Autodesk Inventor part; units mm, degrees
ref_plane "Work Plane4" through (-32.48, 0, 0) normal (1, 0, 0) x (0, 1, 0)
ref_plane "Work Plane5" through (30.48, 0, 0) normal (1, 0, 0) x (0, 1, 0)
ref_plane "XZ Plane" through (0, 0, 0) normal (0, 1, 0) x (-1, 0, 0)
sketch "Sketch1" plane through (0, 0, 0) normal (0, 1, 0) x (-1, 0, 0)
  circle A0 centre (0, 0) radius 30.48
  circle A1 centre (0, 0) radius 32.48
  dimension "d0" = 60.96
  dimension "d2" = 2
extrude "Extrusion1" add sketch "Sketch1" along normal blind 19.05
sketch "Sketch2" plane through (0, 19.05, 0) normal (0, 1, 0) x (1, 0, 0)
  circle A0 centre (0, 0) radius 32.48
  circle A1 centre (0, 0) radius 32.48
extrude "Extrusion2" add sketch "Sketch2" along normal blind 12.7
fillet "Fillet1" radius 6.35 1 edges at (-32.48, 31.75, 0)
sketch "Sketch6" plane through (0, 31.75, 0) normal (0, 1, 0) x (1, 0, 0)
  circle A0 centre (0, 0) radius 3.302
  dimension "d15" = 6.604
extrude "Extrusion5" cut sketch "Sketch6" against normal up to surface (12.7 mm away)
sketch "Sketch10" plane through (0, 0, 0) normal (0, 0, 1) x (1, 0, 0)
  line L0 (-17.78, 19.05) -> (-17.78, -12.7)
  line L1 (-17.78, -12.7) -> (-25.4, -12.7)
  line L2 (-25.4, -12.7) -> (-25.4, 19.05)
  line L3 (-17.78, 19.05) -> (-25.4, 19.05)
  line L4 (-26.13, 31.75) -> (26.13, 31.75)
  line L5 (0, 31.75) -> (0, 0)
  line L6 (32.48, 0) -> (-32.48, 0)
  line L7 (-30.48, 0) -> (-30.48, 19.05)
  line L8 (-17.78, -12.7) -> (-25.4, -8.3006)
  line L9 (-30.48, 19.05) -> (30.48, 19.05)
  point P0 (-30.48, 0)
  point P1 (-25.4, 19.05)
  dimension "d29" = 7.62
  dimension "d33" = 30
  dimension "d42" = 25.4
  dimension "d89" = 31.75
revolve "Revolution2" add sketch "Sketch10" angle 360 about axis through (0, 31.75, 0) along (0, -1, 0) contours L0 L6 L2 L3 | L0 L8 L2 L6
sketch "Sketch11" plane through (0, 0, 0) normal (0, 0, 1) x (1, 0, 0)
  line L0 (25.4, -7.0306) -> (25.4, 25.4)
  circle A0 centre (26.3462, -3.81) radius 2.3813
  circle A1 centre (26.3462, 2.54) radius 2.3813
  line L1 (0, -11.43) -> (0, 31.75)
  line L2 (-26.13, 31.75) -> (26.13, 31.75)
  line L3 (26.3462, 2.54) -> (26.3462, -3.81)
  line L4 (30.48, 19.05) -> (30.48, 0)
  line L5 (30.48, 0) -> (29.972, 19.05)
  line L6 (29.972, 19.05) -> (29.972, 0)
  line L7 (-25.4, -5.08) -> (25.4, -5.08)
  line L8 (-17.78, -12.7) -> (17.78, -12.7)
  point P0 (0, 0)
  point P1 (25.4, -8.3006)
  point P2 (27.772, -0.6806)
  point P3 (17.78, -12.7)
  dimension "d36" = 6.35
  dimension "d37" = 4.7625
  dimension "d38" = 4.7625
  dimension "d43" = 26.3462
  dimension "d91" = 8.89
revolve "Revolution3" cut sketch "Sketch11" angle 360 about axis through (0, -11.43, 0) along (0, 1, 0) contours A0 L7 L0 | L0 A0 | L7 A0 L0 | A1 L0 | L0 A1
sketch "Sketch23" plane through (0, 31.75, 0) normal (0, 1, 0) x (1, 0, 0)
  circle A0 centre (0, 0) radius 5
  dimension "d103" = 10
extrude "Extrusion15" cut sketch "Sketch23" against normal blind 8
ref_plane "Work Plane4" through (-32.48, 0, 0) normal (1, 0, 0) x (0, 1, 0)
sketch "Sketch24" plane through (-32.48, 0, 0) normal (1, 0, 0) x (0, 1, 0)
  circle A0 centre (8.89, 0) radius 1.45
  line L0 (0, -32.48) -> (0, 32.48)
  line L1 (31.75, 5) -> (31.75, -5)
  line L2 (31.75, 0) -> (0, 0) construction
  line L3 (-1.6248, -25.4) -> (-1.6248, 25.4)
  dimension "d106" = 2.9
  dimension "d107" = 8.89
  dimension "d108" = 0
extrude "Extrusion16" cut sketch "Sketch24" along normal up to surface
pattern_circular "Circular Pattern4" count 2 over 360 about axis through (0, 31.75, 0) along (0, -1, 0) of "Extrusion16"
ref_plane "Work Plane5" through (30.48, 0, 0) normal (1, 0, 0) x (0, 1, 0)
sketch "Sketch25" plane through (30.48, 0, 0) normal (1, 0, 0) x (0, 1, 0)
  line L0 (31.75, 5) -> (31.75, -5)
  line L1 (31.75, 0) -> (-12.7, 0)
  line L2 (-12.7, 17.78) -> (-12.7, -17.78)
  line L3 (11.675, -1.6079) -> (8.89, -3.2158)
  line L4 (8.89, -3.2158) -> (6.105, -1.6079)
  line L5 (6.105, -1.6079) -> (6.105, 1.6079)
  line L6 (6.105, 1.6079) -> (8.89, 3.2158)
  line L7 (8.89, 3.2158) -> (11.675, 1.6079)
  line L8 (11.675, 1.6079) -> (11.675, -1.6079)
  line L9 (0, -32.48) -> (0, 32.48)
  circle A0 centre (8.89, 0) radius 1.45
  point P0 (0, 0)
  point P1 (11.675, 0)
  dimension "d115" = 8.89
  dimension "d116" = 2.9
  dimension "d117" = 5.57
extrude "Extrusion17" cut sketch "Sketch25" along normal blind 1.27 and the other way blind 0.635 contours L8 L3 L4 L5 L1 A0 | L1 A0 L5 L6 L7 L8
pattern_circular "Circular Pattern5" count 2 over 360 about axis through (0, 31.75, 0) along (0, -1, 0) of "Extrusion17"
properties part number "Water_Sensor_Cap_3DPrint"
Could you check a few things on this model? Use its own coordinates, in mm. A direction names the side the tool comes from. Round coordinates to 2 decimals unless told otherwise and drop trailing zeros. Loops run counter-clockwise (first coordinate to the right, second up) from the corner with the lowest first, then second, coordinate; pieces in that order, holes last. Notation, with made-up numbers: M 15,52 L 68,52 A25 ccw 68,88 Z; hole C 17,-3.75 d11. An arc over 180 degrees is marked long. Answer as CSV lines item,"result".
1) Imagine slicing it at A-A on y = 14.5. List the corners of the cut face in (x, z) for me.
From the geometry:
outline,"C 0,0 d64.96; C 0,0 d50.8; hole C 0,0 d60.96; hole C 0,0 d35.56"
2) Imagine slicing it at C-C on y = 21. List the corners of the cut face in (x, z) for me.
From the geometry:
outline,"C 0,0 d64.96; hole C 0,0 d6.6"
3) Which directions (+Z, -Z, +X, -X, +Y, -Y) give clear straight access to the entire face, cutting with the end or side of a thin tool? Please do faces 4 (the cylindrical face through (5.506, 11.988, -24.796)), 5 (the cylindrical face through (32.12, 7.44, 0.06)), 6 (the flat face through (-31.02, 7.48, -2.4)), 7 (the flat face through (3.3, 23.75, -1.2)).
From the geometry:
face 4,"-Y"
face 5,"+X"
face 6,"none"
face 7,"+Y"
4) We'd pull the mould along X, two halves only. Please class faces 1 (the cylindrical face through (5.506, -7.132, -24.796)), 2 (the flat face through (5.4, 31.75, -0.4)), 3 (the flat face through (31.75, 8.2, 1.5)): released by +X, released by -X, zero draft, split by the parting line, or undercut.
From the geometry:
face 1,"split by the parting line"
face 2,"zero draft"
face 3,"undercut"
5) If I drill on probe 1 along Z at (x, y) = (0.5, 8); probe 2 along X at (y, z) = (6.5, 0); probe 3 along Z at (x, y) = (18.5, 1.5), over which ranges is the centre line in solid material (lowest first)?
From the geometry:
probe 1,"-32.48 to -30.48, -25.4 to -17.77, 17.77 to 25.4, 30.48 to 32.48"
probe 2,"-32.48 to -31.75, -25.4 to -17.78, 17.78 to 25.4, 31.75 to 32.48"
probe 3,"-26.7 to -24.22, -15.61 to 15.61, 24.22 to 26.7"
6) Imagine slicing it at D-D on y = 2. List the corners of the cut face in (x, z) for me, and give its area (3 significant figures).
From the geometry:
outline,"C 0,0 d64.96; C 0,0 d48.05; hole C 0,0 d60.96; hole C 0,0 d35.56"
area,"1,220 mm^2"
7) For pin 1 Ø4 at (y, z) = (-2.5, -12) entering from +X; pin 2 Ø8 at (x, z) = (-1.5, -2) entering from +Y; pin 3 Ø6 at (y, z) = (13, 23) entering from +X; pin 4 Ø4 at (x, y) = (-22, -4.5) entering from -Z, each with a flat end and sliding along its axis, tell me the tip position at first contact or that it passes through.
From the geometry:
pin 1,"x = 23.26"
pin 2,"y = 31.75"
pin 3,"x = 25.59"
pin 4,"z = -14.76"
